```python
from build123d import *

# Parameters (mm, degrees)
SKETCH1_W               = 40
SKETCH1_H               = 40
BOSS_EXTRUDE1_DEPTH     = 20
CUT_EXTRUDE2_DEPTH      = 35.641016151
CUT_EXTRUDE2_DEPTH_BACK = 35.641016151
SKETCH2_R               = 12.5


with BuildPart() as part:
    # Sketch1 → Boss-Extrude1 (new, symmetric)
    with BuildSketch(Plane.XY):
        Rectangle(SKETCH1_W, SKETCH1_H)
    extrude(amount=BOSS_EXTRUDE1_DEPTH, both=True)

    # Sketch2 → Cut-Extrude2 (cut, two sides: drawn at the far end of the back side and taken through both)
    with BuildSketch(Plane.ZX.offset(-CUT_EXTRUDE2_DEPTH_BACK)):
        Circle(SKETCH2_R)
    extrude(amount=CUT_EXTRUDE2_DEPTH + CUT_EXTRUDE2_DEPTH_BACK, mode=Mode.SUBTRACT)


solid = part.part
```
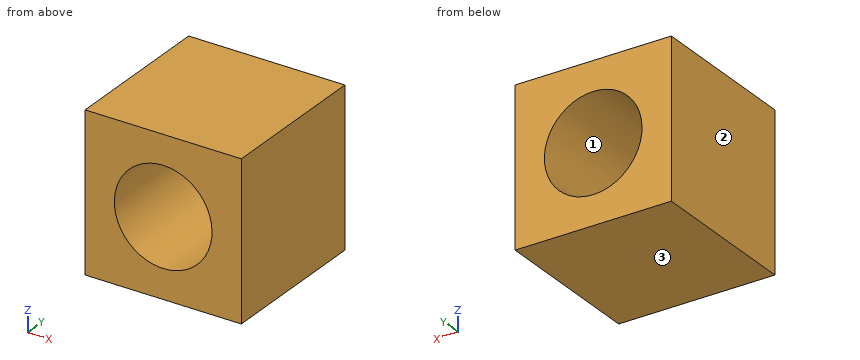
Model file for the job. Use its own axes, mm. Face numbers are marked on the shaded views. Coordinates: 2 decimals unless noted, no trailing zeros. Order: outer loops, then holes, each group sorted by start corner. A loop starts at its lowest first (then second) coordinate and runs counter-clockwise, first axis right, second up. Notation, with made-up numbers: (-18.75, 88.5) -> (1.25, 88.5) arc R11 cw to (1.25, 107.5) -> close; hole circle Ø3 at (35.25, -20.75). An arc over 180 degrees is marked (long way). Return JSON: item names as keys, results as strings.
Item 1: Slice it at A-A (x = 0). Write the cut outline in (y, z), then the cut area to 3 significant figures.
Model answer:
{"outline": "(-20, -20) -> (20, -20) -> (20, -12.5) -> (-20, -12.5) -> close; (-20, 12.5) -> (20, 12.5) -> (20, 20) -> (-20, 20) -> close", "area": "600 mm²"}
Item 2: Slice it at B-B (z = 0). Write the cut outline in (x, y).
Model answer:
{"outline": "(-20, -20) -> (-12.5, -20) -> (-12.5, 20) -> (-20, 20) -> close; (12.5, -20) -> (20, -20) -> (20, 20) -> (12.5, 20) -> close"}
Item 3: Slice it at C-C (y = 12.5). Write the cut outline in (x, z).
Model answer:
{"outline": "(-20, -20) -> (20, -20) -> (20, 20) -> (-20, 20) -> close; hole circle Ø25 at (0, 0)"}
Item 4: Wall check: line 1 along Z through (x, y) = (0, -12); line 2 along X through (y, z) = (14, -8). Give the ranges that are in metal, low to high. Write a range as from..to.
Model answer:
{"line 1": "z = -20..-12.5, 12.5..20", "line 2": "x = -20..-9.6, 9.6..20"}
Item 5: Pin check, flat tip, straight feed: P1, Ø4, axis at x = 8.5, z = 3, coming from the +Y side. Stop position of the tip, or through.
Model answer:
{"P1": "passes through"}
Item 6: Mould opens along X. For the marked faces 1, 2 and 3 say: pulls with the +X half, pulls with the -X half, needs draft (parallel to the pull), parting line crosses it, or undercut.
Model answer:
{"face 1": "undercut", "face 2": "pulls with the -X half", "face 3": "needs draft"}
